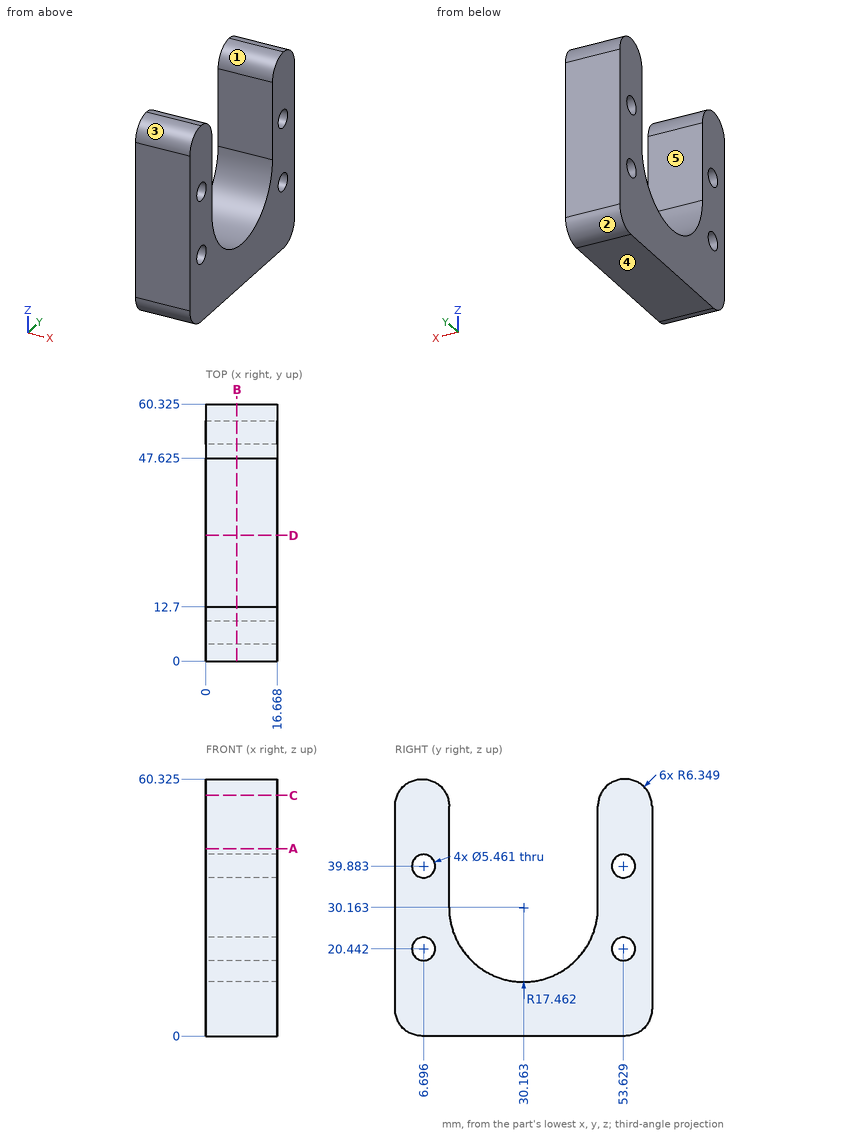
Can you work these out from the drawing? Everything is in mm from the part's minimum corner. A direction names the side the tool comes from. Coordinates: 2 decimals unless noted, no trailing zeros. Write each loop counter-clockwise with the first axis right and the second up, starting at its lowest first coordinate (ties: lowest second). Pieces come first, ordered by that corner, then holes. Notation, with made-up numbers: (83.5, 43.5) - (122.5, 43.5) arc R18 ccw to (122.5, 48.5) - close; hole circle Ø11 at (-23, 28.5). An arc over 180 degrees is marked (long way). Use a Markdown table: item, result.
Q1. Please list where these lines run through material, in increasing order: L1, parallel to Y at x = 4.25, z = 29.5 (1 decimal); L2, parallel to Z at x = 2.5, y = 5 (1 decimal); L3, parallel to Z at x = 4.25, y = 55 (1 decimal).
Geometry check:
| item | result |
|---|---|
| L1 | y = 0 to 12.7, 47.6 to 60.3 |
| L2 | z = 0.1 to 18.3, 22.6 to 37.7, 42 to 60.2 |
| L3 | z = 0.1 to 18.1, 22.8 to 37.5, 42.2 to 60.2 |
Q2. Which directions (+Z, -Z, +X, -X, +Y, -Y) give clear straight access to the entire face, cutting with the end or side of a thin tool? Please do the marked faces 4 and 5.
Geometry check:
| item | result |
|---|---|
| face 4 | -Z, +X, -X, +Y, -Y |
| face 5 | +Z, +X, -X |
Q3. I'm going to push a flat-ended pin straight in: pin 1 Ø1.5 at (x, y) = (7, 39.5) entering from +Z. Where does the tip first touch, or does it pass through?
Geometry check:
| item | result |
|---|---|
| pin 1 | stops at z = 15.91 |
Q4. Imagine slicing it at B-B (x = 7.25). Count the separate pieces of the cut face and the enclosed holes in it, and give its area (3 significant figures).
Geometry check:
| item | result |
|---|---|
| separate pieces | 1 |
| enclosed holes | 4 |
| area | 1,960 mm2 |
Q5. Thinking about a two-plate mould opening in Y: for the marked faces 1, 2 and 3, which applies, +Y half, -Y half, draft (parallel to the pull), parting line (faces both ways), or undercut?
Geometry check:
| item | result |
|---|---|
| face 1 | undercut |
| face 2 | +Y half |
| face 3 | -Y half |
Q6. Imagine slicing it at D-D (y = 29.5). List the corners of the cut face in (x, z) for me.
Geometry check:
| item | result |
|---|---|
| outline | (0, 0) - (16.67, 0) - (16.67, 12.71) - (0, 12.71) - close |
Q7. Imagine slicing it at A-A (z = 44). List the corners of the cut face in (x, y) for me (1 decimal), and give its area (3 significant figures).
Geometry check:
| item | result |
|---|---|
| outline | (0, 0) - (16.7, 0) - (16.7, 12.7) - (0, 12.7) - close; (0, 47.6) - (16.7, 47.6) - (16.7, 60.3) - (0, 60.3) - close |
| area | 423 mm2 |
Q8. Imagine slicing it at C-C (z = 56.5). List the corners of the cut face in (x, y) for me.
Geometry check:
| item | result |
|---|---|
| outline | (0, 0.52) - (16.67, 0.52) - (16.67, 12.18) - (0, 12.18) - close; (0, 48.15) - (16.67, 48.15) - (16.67, 59.8) - (0, 59.8) - close |
